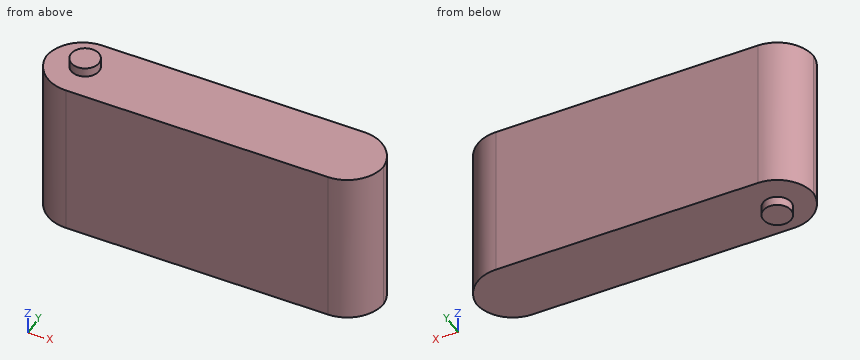
from build123d import *

# Parameters (mm, degrees)
F0_W        = 72
F0_H        = 34
F1_DEPTH    = 15
F2_T1_DEPTH = 74
F3_R        = 3
F4_DEPTH    = 2
F5_R        = 3
F6_DEPTH    = 2


# Not quite as in the source:
# - a fillet or chamfer that OpenCascade refuses, or shapes differently, is made with other operations: its cross-section is extruded or revolved along the edge and cut away or added


with BuildPart() as f1:
    # F0 (on Front) → F1 (new body)
    with BuildSketch(Plane.XZ):
        Rectangle(F0_W, F0_H)
    extrude(amount=F1_DEPTH)

    # F2: fillet of radius 8 on 4 edges, made by hand

    # F2_s2 → F2_t1 (cut)
    with BuildSketch(Plane.XY.offset(-37)):
        with BuildLine():
            ThreePointArc((-36, -8), (-33.6568542495, -2.3431457505), (-28, 0))
            Line((-28, 0), (-36, 0))
            Line((-36, 0), (-36, -8))
        make_face()
        with BuildLine():
            ThreePointArc((-36, -7), (-33.6568542495, -12.6568542495), (-28, -15))
            Line((-28, -15), (-36, -15))
            Line((-36, -15), (-36, -7))
        make_face()
        with BuildLine():
            ThreePointArc((36, -7), (33.6568542495, -12.6568542495), (28, -15))
            Line((28, -15), (36, -15))
            Line((36, -15), (36, -7))
        make_face()
        with BuildLine():
            ThreePointArc((36, -8), (33.6568542495, -2.3431457505), (28, 0))
            Line((28, 0), (36, 0))
            Line((36, 0), (36, -8))
        make_face()
    extrude(amount=F2_T1_DEPTH, mode=Mode.SUBTRACT)

    # F3 (on face) → F4 (join)
    with BuildSketch(Plane.XY.offset(17)):
        with Locations((-28, -7)):
            Circle(F3_R)
    extrude(amount=F4_DEPTH)

    # F5 (on face) → F6 (join)
    with BuildSketch(Plane(origin=(0, 0, -17), x_dir=(1, 0, 0), z_dir=(0, 0, -1))):
        with Locations((-28, 8)):
            Circle(F5_R)
    extrude(amount=F6_DEPTH)


solid = f1.part
Here's how the part is built. I have some questions about the finished solid (model axes, mm). Coordinates: 2 decimals unless noted, no trailing zeros. Write each loop counter-clockwise with the first axis right and the second up, starting at its lowest first coordinate (ties: lowest second). Pieces come first, ordered by that corner, then holes.
Item 1: If I drill on line 1 (Z direction, x = -6, y = -12.25); line 2 (X direction, y = -4.75, z = 14.5); line 3 (X direction, y = -8, z = 16), over which ranges is the centre line in solid material (lowest first)?
Item 2: I want a section at D-D on y = -1.25. Write out the boundary of the cut face in (x, z).
Item 3: I want a section at B-B on x = -2.5. Write out the boundary of the cut face in (y, z), and give its area (3 significant figures).
Item 4: I want a section at A-A on z = 15.5. Write out the boundary of the cut face in (x, y), and give its area (3 significant figures).
Item 5: Will these pins go through, and if not, where does the flat tip stop? pin 1 (8 mm diameter, centred on y = -4.5, z = 12.5, fed in from -X); pin 2 (6 mm diameter, centred on y = -2, z = -7.5, fed in from +X); pin 3 (4.5 mm diameter, centred on x = -3.5, y = -10, fed in from -Z); pin 4 (7.5 mm diameter, centred on x = 18, y = -7, fed in from +Z).
Item 6: I want a section at C-C on y = -8.75. Write out the boundary of the cut face in (x, z), and give its area (3 significant figures).
Findings below:
1. line 1: z = -17 to 17
1. line 2: x = -35.31 to 35.31
1. line 3: x = -35.94 to 35.94
2. outline: (-32.29, -17) - (32.29, -17) - (32.29, 17) - (-32.29, 17) - close
3. outline: (-15, -17) - (0, -17) - (0, 17) - (-15, 17) - close
3. area: 510 mm2
4. outline: (-35.98, -7.5) arc R8 ccw to (-28, -15) - (28, -15) arc R8 ccw to (35.98, -7.5) arc R8 ccw to (28, 0) - (-28, 0) arc R8 ccw to start
4. area: 1,030 mm2
5. pin 1: stops at x = -35.98
5. pin 2: stops at x = 35.42
5. pin 3: stops at z = -17
5. pin 4: stops at z = 17
6. outline: (-35.81, -17) - (-30.9, -17) - (-30.9, -19) - (-25.1, -19) - (-25.1, -17) - (35.81, -17) - (35.81, 17) - (-25.56, 17) - (-25.56, 19) - (-30.44, 19) - (-30.44, 17) - (-35.81, 17) - close
6. area: 2,460 mm2
